Part model, mm, in its own coordinate system. A direction names the side the tool comes from. Round coordinates to 2 decimals unless told otherwise and drop trailing zeros. Loops run counter-clockwise (first coordinate to the right, second up) from the corner with the lowest first, then second, coordinate; pieces in that order, holes last. Notation, with made-up numbers: M -3.75,14 L 13.25,14 A36 cw 13.25,49 Z; hole C -25.75,-26 d9. An arc over 180 degrees is marked long. Put each result on its own line as item: value. Start each with the question number.
```python
from build123d import *

# Parameters (mm, degrees)
F0_R      = 8.3502
F1_DEPTH  = 33.02
F2_W      = 6.7056
F2_H      = 26.9042
F3_DEPTH  = 76.2
F4_W      = 20.8406
F4_H      = 41.44
F4_R      = 2.032
F5_DEPTH  = 25.4
F6_W      = 7.7596
F6_H      = 5.3483209641
F7_DEPTH  = 25.4
F8_R      = 0.4
F9_W      = 27.051
F9_H      = 26.9042
F10_DEPTH = 12.7
F11_W     = 3.81
F11_H     = 12.7
F11_R     = 1.524
F12_DEPTH = 14.7828
F13_DEPTH = 12.7
F14_W     = 2.88544
F14_H     = 6.6294
F15_DEPTH = 26.9052


with BuildPart() as f1:
    # F0 (on Top) → F1 (new body)
    with BuildSketch(Plane.XY):
        with BuildLine():
            Line((25.4, 13.4521), (0, 13.4521))
            ThreePointArc((0, 13.4521), (-13.4521, 0), (0, -13.4521))
            Line((0, -13.4521), (25.4, -13.4521))
            Line((25.4, -13.4521), (25.4, 13.4521))
        make_face()
        Circle(F0_R, mode=Mode.SUBTRACT)
    extrude(amount=F1_DEPTH)

    # F2 (on face) → F3 (join)
    with BuildSketch(Plane.XY.offset(33.02)):
        with Locations((22.0472, 0)):
            Rectangle(F2_W, F2_H)
    extrude(amount=F3_DEPTH)

    # F4 (on face) → F5 (cut)
    with BuildSketch(Plane(origin=(18.6944, 0, 0), x_dir=(0, -1, 0), z_dir=(-1, 0, 0))):
        with Locations((0, 80.55)):
            Rectangle(F4_W, F4_H)
        with Locations((-5.0165, 104.934)):
            Circle(F4_R)
        with Locations((-5.0165, 56.166)):
            Circle(F4_R)
        with Locations((5.0165, 56.166)):
            Circle(F4_R)
        with Locations((5.0165, 104.934)):
            Circle(F4_R)
    extrude(amount=-F5_DEPTH, mode=Mode.SUBTRACT)

    # F6 (on face) → F7 (cut)
    with BuildSketch(Plane(origin=(18.6944, 0, 0), x_dir=(0, -1, 0), z_dir=(-1, 0, 0))):
        with Locations((0, 103.944160482)):
            Rectangle(F6_W, F6_H)
    extrude(amount=-F7_DEPTH, mode=Mode.SUBTRACT)

    # F8
    f8_edges = [f1.edges().sort_by_distance(p)[0] for p in [
        (22.0472, 3.8798, 103.249679),
        (22.0472, -3.8798, 103.249679),
        (22.0472, 3.8798, 101.27),
        (22.0472, -3.8798, 101.27),
        (22.0472, 3.8798, 106.618321),
        (22.0472, -3.8798, 106.618321),
    ]]
    fillet(f8_edges, radius=F8_R)

    # F9 (on face) → F10 (join)
    with BuildSketch(Plane.XY.offset(109.22)):
        with Locations((11.8745, 0)):
            Rectangle(F9_W, F9_H)
    extrude(amount=F10_DEPTH)

    # F11 (on face) → F12 (cut)
    with BuildSketch(Plane(origin=(-1.651, 0, 0), x_dir=(0, -1, 0), z_dir=(-1, 0, 0))):
        with Locations((0, 115.57)):
            Rectangle(F11_W, F11_H)
        with Locations((-10.414, 115.57)):
            Circle(F11_R)
        with Locations((10.414, 115.57)):
            Circle(F11_R)
    extrude(amount=-F12_DEPTH, mode=Mode.SUBTRACT)

    # F13 (cut): faces of the model
    f13_faces = [f1.faces().sort_by_distance(p)[0] for p in [
        (13.1318, 10.414, 115.57),
        (13.1318, -10.414, 115.57),
    ]]
    extrude(f13_faces, amount=-F13_DEPTH, mode=Mode.SUBTRACT)

    # F14 (on face) → F15 (cut, through all)
    with BuildSketch(Plane(origin=(0, 13.4521, 0), x_dir=(-1, 0, 0), z_dir=(0, 1, 0))):
        with Locations((-4.23672, 115.57)):
            Rectangle(F14_W, F14_H)
    extrude(amount=-F15_DEPTH, mode=Mode.SUBTRACT)


solid = f1.part
```
1. Cut at D-D, the plane z = 115.57. Give the number of separate pieces and of enclosed holes in the cut face, and give its area (3 significant figures).
2. Mould opens along X. For faces 4 (the flat face through (4, -8, 118.885)), 5 (the flat face through (21, 13.452, 47)), 6 (the flat face through (-1.651, -8, 115)) say: released by +X, released by -X, zero draft, split by the parting line, or undercut.
3. Cut at A-A, the plane x = 14.5. Give the cut face in (y, z).
4. Drop flat-ended pins along their axis: pin 1 (12.5 mm diameter, centred on y = -7, z = 113, fed in from -X); pin 2 (2.5 mm diameter, centred on y = -5.02, z = 104.93, fed in from -X); pin 3 (3 mm diameter, centred on x = 14, y = 10, fed in from -Z); pin 4 (0.9 mm diameter, centred on x = 3.5, y = 5.5, fed in from -Z). Give the stop position or say it passes through.
5. Cut at C-C, the plane x = 1.5. Give the cut face in (y, z) (3 decimals).
6. Wall check: L1, parallel to Y at x = 16, z = 115.57; L2, parallel to Z at x = 4, y = 8; L3, parallel to Z at x = 11, y = -5. Give the ranges that are in metal, low to high.
7. Which spindle directions (+Z, -Z, +X, -X, +Y, -Y) get a long thin tool onto all of the face, cutting with end or side? Do faces 1 (the flat face through (2.794, 8, 116)), 2 (the flat face through (22, -7, 101.27)), 3 (the flat face through (-1.651, 8, 115)). Say none if no direction does.
8. Cut at B-B, the plane z = 80.5. Give the cut face in (x, y).
Results list:
1. separate pieces: 7
1. enclosed holes: 0
1. area: 458 mm^2
2. face 4: undercut
2. face 5: zero draft
2. face 6: released by -X
3. outline: M -13.45,0 L 13.45,0 L 13.45,33.02 L -13.45,33.02 Z; M -13.45,109.22 L 13.45,109.22 L 13.45,121.92 L -13.45,121.92 Z; hole C -10.41,115.57 d3.05; hole C 10.41,115.57 d3.05
4. pin 1: stops at x = -1.65
4. pin 2: passes through
4. pin 3: stops at z = 0
4. pin 4: stops at z = 109.22
5. outline: M -13.452,0 L -8.214,0 L -8.214,33.02 L -13.452,33.02 Z; M -13.452,109.22 L -1.905,109.22 L -1.905,121.92 L -13.452,121.92 Z; M 1.905,109.22 L 13.452,109.22 L 13.452,121.92 L 1.905,121.92 Z; M 8.214,0 L 13.452,0 L 13.452,33.02 L 8.214,33.02 Z; hole C -10.414,115.57 d3.048; hole C 10.414,115.57 d3.048
6. L1: y = -13.45 to -11.94, -8.89 to 8.89, 11.94 to 13.45
6. L2: z = 0 to 33.02, 109.22 to 112.26, 118.88 to 121.92
6. L3: z = 0 to 33.02, 109.22 to 121.92
7. face 1: +Y, -Y
7. face 2: +X, -X
7. face 3: +Z, -X, +Y, -Y
8. outline: M 18.69,-13.45 L 25.4,-13.45 L 25.4,-10.42 L 18.69,-10.42 Z; M 18.69,10.42 L 25.4,10.42 L 25.4,13.45 L 18.69,13.45 Z
